Autodesk Inventor part; units mm, degrees
ref_plane "YZ Plane" through (0, 0, 0) normal (1, 0, 0) x (0, 1, 0)
ref_plane "XZ Plane" through (0, 0, 0) normal (0, 1, 0) x (-1, 0, 0)
ref_plane "XY Plane" through (0, 0, 0) normal (0, 0, 1) x (1, 0, 0)
sketch "Sketch1" plane through (0, 0, 0) normal (0, 1, 0) x (-1, 0, 0)
  circle A0 centre (0, 0) radius 20
  dimension "d0" = 40
extrude "Extrusion1" add sketch "Sketch1" along normal blind 27
sketch "Sketch2" plane through (0, 27, 0) normal (0, 1, 0) x (1, 0, 0)
  circle A0 centre (0, 0) radius 20 construction
  circle A1 centre (0, 0) radius 20 construction
  line L0 (0, -20) -> (0, 20) construction
  arc A2 (0, -20) -> (0, 20) centre (0, 0) ccw
  line L1 (0, -20) -> (0, 20)
  dimension "d3" = 40
revolve "Revolution1" add sketch "Sketch2" angle 180 about axis through (0, 27, 20) along (0, 0, 1)
sketch "Sketch3" plane through (0, 0, 0) normal (0, 0, 1) x (1, 0, 0)
  line L0 (20, 27) -> (-20, 27) construction
  line L1 (20, 27) -> (-20, 27) construction
  line L2 (20, 0) -> (-20, 0) construction
  circle A0 centre (0, 27) radius 5
  arc A1 (20, 27) -> (-20, 27) centre (0, 27) ccw construction
  point P0 (0, 0)
  point P1 (0, 0)
  dimension "d5" = 10
extrude "Extrusion2" cut sketch "Sketch3" along normal through all both and the other way through all
sketch "Sketch4" plane through (0, 0, 0) normal (1, 0, 0) x (0, 1, 0)
  line L0 (27, 19.3649) -> (27, 19.3649) construction
  line L1 (27, 19.3649) -> (27, -19.3649) construction
  line L2 (27, -19.3649) -> (27, -19.3649) construction
  line L3 (27, -19.3649) -> (27, 19.3649) construction
  line L4 (27, 19.3649) -> (27, 19.3649) construction
  line L5 (27, -19.3649) -> (27, -19.3649) construction
  line L6 (0, -20) -> (0, 20) construction
  line L7 (27, -19.3649) -> (27, 19.3649) construction
  line L8 (27, 19.3649) -> (27, -19.3649) construction
  line L9 (27, -19.3649) -> (27, 19.3649) construction
  arc A0 (27, 6) -> (27, -6) centre (27, 0) ccw
  line L10 (27, -6) -> (47.2684, -6)
  line L11 (27, 6) -> (47.2684, 6)
  line L12 (47.2684, -6) -> (47.2684, 6)
  point P0 (0, 0)
  dimension "d8" = 12
  dimension "d9" = 20.2684
extrude "Extrusion3" cut sketch "Sketch4" along normal through all both and the other way through all
sketch "Sketch5" plane through (0, 0, 0) normal (0, -1, 0) x (1, 0, 0)
  circle A0 centre (0, 0) radius 10
  dimension "d12" = 20
extrude "Extrusion4" cut sketch "Sketch5" against normal up to surface (27 mm away)
properties part number "cupula_obj5"
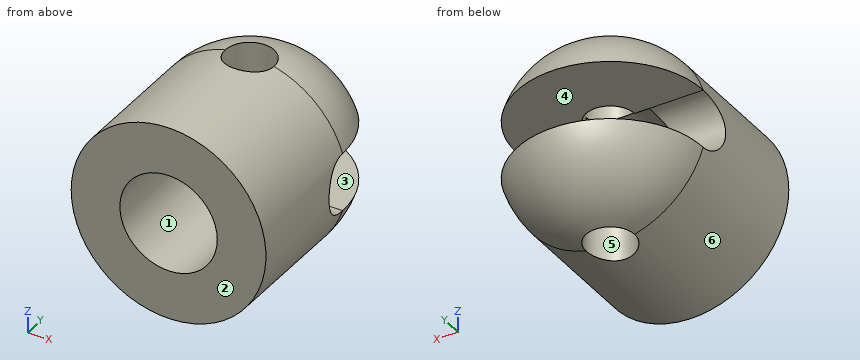
Verification items for the finished model (mm, model axes). Face numbers are marked on the shaded views. A direction names the side the tool comes from. Coordinates: 2 decimals unless noted, no trailing zeros. Write each loop counter-clockwise with the first axis right and the second up, starting at its lowest first coordinate (ties: lowest second). Pieces come first, ordered by that corner, then holes. Notation, with made-up numbers: (20.25, 18) - (74.25, 18) arc R29 cw to (74.25, 56) - close; hole circle Ø6 at (18.5, 12). An arc over 180 degrees is marked (long way). One line per question, with ' | ' between items. Start each with the question number.
1. Draft check along Z on the marked faces 4, 5 and 6. Enter one of: released by +Z, released by -Z, zero draft, split by the parting line, or undercut.
2. Section check A-A (x = 0). Enter the section's corners in (y, z).
3. Access from +Z, -Z, +X, -X, +Y, -Y to the whole of each face (thin tool, end or side, straight path). Record for the marked faces 1, 2 and 3.
4. Section check C-C (z = -8). Enter the section's corners in (x, y).
5. Section check B-B (z = 0). Enter the section's corners in (x, y), plus the area to 3 significant figures.
6. Gauge pin test, flat ends, axial feed: P1, Ø1.5, axis at x = -14, y = 22.5, coming from the +Z side; P2, Ø15.5, axis at x = -3, y = 35, coming from the +Z side; P3, Ø4, axis at y = 35, z = 12.5, coming from the -X side. Record the tip position at first contact, or that the pin passes through.
7. Material ranges on line 1 along X through (y, z) = (9, 0); line 2 along Z through (x, y) = (-3, 38), recorded low to high.
8. Section check D-D (x = 16). Enter the section's corners in (y, z).
Computed values:
1) face 4: undercut | face 5: zero draft | face 6: split by the parting line
2) outline: (0, -20) - (22, -20) - (22, -10) - (0, -10) - close; (0, 10) - (22, 10) - (22, 20) - (0, 20) - close; (32, -19.36) arc R20 ccw to (46.08, -6) - (32, -6) - close; (32, 6) - (46.08, 6) arc R20 ccw to (32, 19.36) - close
3) face 1: -Y | face 2: +Z, -Z, +X, -X, -Y | face 3: +X, -X, +Y
4) outline: (-18.33, 0) - (-6, 0) - (-6, 27) - (-5, 27) arc R5 cw to (5, 27) - (6, 27) - (6, 0) - (18.33, 0) - (18.33, 27) arc R18.33 ccw to (-18.33, 27) - close
5) outline: (-20, 0) - (-10, 0) - (-10, 21) - (-20, 21) - close; (10, 0) - (20, 0) - (20, 21) - (10, 21) - close | area: 420 mm²
6) P1: z = 14.98 | P2: z = 19.36 | P3: x = -15.33
7) line 1: -20 to -10, 10 to 20 | line 2: -16.43 to -6, 6 to 16.43
8) outline: (0, -12) - (27, -12) arc R12 ccw to (37.39, -6) - (27, -6) arc R6 cw to (27, 6) - (37.39, 6) arc R12 ccw to (27, 12) - (0, 12) - close
